Source: CAD feature listing. Evaluate the final solid. Frame: model axes, mm. Round coordinates to 2 decimals unless told otherwise and drop trailing zeros. Order: outer loops, then holes, each group sorted by start corner. A loop starts at its lowest first (then second) coordinate and runs counter-clockwise, first axis right, second up. Notation, with made-up numbers: (60.5, 61.5) - (70.5, 61.5) arc R31 ccw to (70.5, 98.5) - close; hole circle Ø5 at (-29, -19.75). An arc over 180 degrees is marked (long way). Use one line per item in the form item = value. Start each with the question number.
Q1. Cut plane A-A, the plane y = -3.25. Return the cut outline in (x, z).
Q2. Pin query (flat end, axial travel): pin 1 Ø5 at (x, z) = (0, -155) entering from +Y. Return the tip coordinate at first contact, or that it passes through.
Q3. Ray query, line 1 (Y direction, x = 7.5, z = -32); line 2 (X direction, y = 9.4, z = 155). Return the intervals inside material, ascending. Write a range as [from, to].
Q4. Cut plane B-B, the plane z = -68. Return the cut outline in (x, y).
from build123d import *

# Parameters (mm, degrees)
SKETCH_1_W            = 20
SKETCH_1_H            = 20
SKETCH_1_W_2          = 18
SKETCH_1_H_2          = 18
EXTRUDE_1_DEPTH       = 165
MM_1_D                = 4
HOLE_WIZARD_4_0_4_1_D = 4
HOLE_WIZARD_4_0_4_2_D = 4


with BuildPart() as part:
    # 草图1 → 凸台-拉伸1 (new, symmetric)
    with BuildSketch(Plane.XY):
        Rectangle(SKETCH_1_W, SKETCH_1_H)
        Rectangle(SKETCH_1_W_2, SKETCH_1_H_2, mode=Mode.SUBTRACT)
    extrude(amount=EXTRUDE_1_DEPTH, both=True)

    # 大小mm 暗销孔1 (through all)
    with Locations(Plane(origin=(0, -10, 0), x_dir=(-1, 0, 0), z_dir=(0, -1, 0))):
        with Locations((0, -107.3)):
            mm_1 = Hole(MM_1_D / 2)

    # 镜向1: 大小mm 暗销孔1 across plane
    add(mm_1.mirror(Plane.XY), mode=Mode.SUBTRACT)

    # Ø4.0 (4) 直径孔1 (through all)
    with Locations(Plane(origin=(0, -10, 0), x_dir=(-1, 0, 0), z_dir=(0, -1, 0))):
        with Locations((0, -155)):
            hole_wizard_4_0_4_1 = Hole(HOLE_WIZARD_4_0_4_1_D / 2)

    # 镜向2: Ø4.0 (4) 直径孔1 across plane
    add(hole_wizard_4_0_4_1.mirror(Plane.XY), mode=Mode.SUBTRACT)

    # Ø4.0 (4) 直径孔2 (through all)
    with Locations(Plane(origin=(0, -10, 0), x_dir=(-1, 0, 0), z_dir=(0, -1, 0))):
        with Locations((0, -90), (0, 0)):
            Hole(HOLE_WIZARD_4_0_4_2_D / 2)


solid = part.part
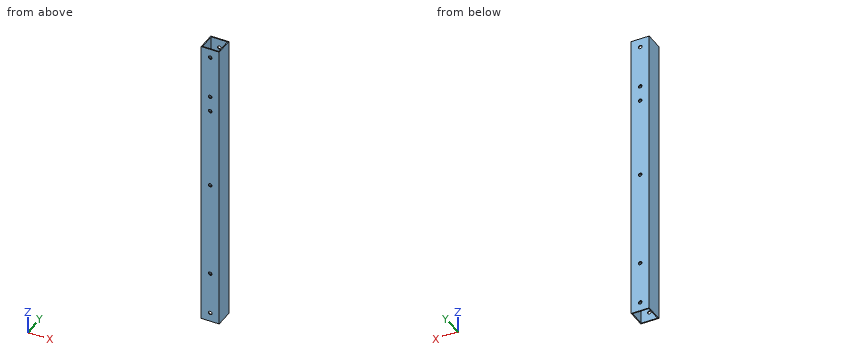
Completed:
q1.outline = (-10, -165) - (-9, -165) - (-9, 165) - (-10, 165) - close; (9, -165) - (10, -165) - (10, 165) - (9, 165) - close
q2.pin_1 = 10
q3.line_1 = [-10, -9], [9, 10]
q3.line_2 = [-10, -2], [2, 10]
q4.outline = (-10, -10) - (10, -10) - (10, 10) - (-10, 10) - close; hole (-9, -9) - (9, -9) - (9, 9) - (-9, 9) - close
